```python
from build123d import *

# Parameters (mm, degrees)
F0_W      = 450
F0_H      = 450
F1_DEPTH  = 50
F2_W      = 40
F2_H      = 40
F3_DEPTH  = 400
F4_W      = 40
F4_H      = 40
F5_DEPTH  = 400
F6_W      = 40
F6_H      = 40
F7_DEPTH  = 400
F8_W      = 40
F8_H      = 40
F9_DEPTH  = 400
F10_W     = 450
F10_H     = 50
F11_DEPTH = 450
F13_DEPTH = 450
F15_DEPTH = 450.001
F17_DEPTH = 450.001
F18_DEPTH = 100
F19_DEPTH = 100
F20_DEPTH = 200
F21_DEPTH = 200


with BuildPart() as f1:
    # F0 (on Top) → F1 (new body)
    with BuildSketch(Plane.XY):
        with Locations((225, 225)):
            Rectangle(F0_W, F0_H)
    extrude(amount=F1_DEPTH)

    # F2 (on face) → F3 (join)
    with BuildSketch(Plane(origin=(0, 0, 0), x_dir=(1, 0, 0), z_dir=(0, 0, -1))):
        with Locations((20, -430)):
            Rectangle(F2_W, F2_H)
    extrude(amount=F3_DEPTH)

    # F4 (on face) → F5 (join)
    with BuildSketch(Plane(origin=(0, 0, 0), x_dir=(1, 0, 0), z_dir=(0, 0, -1))):
        with Locations((20, -20)):
            Rectangle(F4_W, F4_H)
    extrude(amount=F5_DEPTH)

    # F6 (on face) → F7 (join)
    with BuildSketch(Plane(origin=(0, 0, 0), x_dir=(1, 0, 0), z_dir=(0, 0, -1))):
        with Locations((430, -430)):
            Rectangle(F6_W, F6_H)
    extrude(amount=F7_DEPTH)

    # F8 (on face) → F9 (join)
    with BuildSketch(Plane(origin=(0, 0, 0), x_dir=(1, 0, 0), z_dir=(0, 0, -1))):
        with Locations((430, -20)):
            Rectangle(F8_W, F8_H)
    extrude(amount=F9_DEPTH)

    # F10 (on face) → F11 (join)
    with BuildSketch(Plane.XY.offset(50)):
        with Locations((225, 425)):
            Rectangle(F10_W, F10_H)
    extrude(amount=F11_DEPTH)

    # F12 (on face) → F13 (cut)
    with BuildSketch(Plane.YZ.offset(450)):
        Polygon((400, 500), (400, 50), (430, 500), align=None)
    extrude(amount=-F13_DEPTH, mode=Mode.SUBTRACT)

    # F14 (on face) → F15 (cut, through all)
    with BuildSketch(Plane(origin=(0, 0, 0), x_dir=(0, -1, 0), z_dir=(-1, 0, 0))):
        Polygon((-410, -400), (-410, 0), (-430, -400), align=None)
    extrude(amount=-F15_DEPTH, mode=Mode.SUBTRACT)

    # F16 (on face) → F17 (cut, through all)
    with BuildSketch(Plane(origin=(0, 0, 0), x_dir=(0, -1, 0), z_dir=(-1, 0, 0))):
        Polygon((-20, -400), (-40, 0), (-40, -400), align=None)
    extrude(amount=-F17_DEPTH, mode=Mode.SUBTRACT)

    # F18 (add): a face of the model
    f18_faces = [f1.faces().sort_by_distance(p)[0] for p in [
        (225, 200, 50),
    ]]
    extrude(f18_faces, amount=F18_DEPTH)

    # F19 (cut): a face of the model
    f19_faces = [f1.faces().sort_by_distance(p)[0] for p in [
        (225, 200, 150),
    ]]
    extrude(f19_faces, amount=-F19_DEPTH, mode=Mode.SUBTRACT)

    # F20 (add): a face of the model
    f20_faces = [f1.faces().sort_by_distance(p)[0] for p in [
        (225, 200, 50),
    ]]
    extrude(f20_faces, amount=F20_DEPTH)

    # F21 (cut): a face of the model
    f21_faces = [f1.faces().sort_by_distance(p)[0] for p in [
        (225, 200, 250),
    ]]
    extrude(f21_faces, amount=-F21_DEPTH, mode=Mode.SUBTRACT)


solid = f1.part
```
Verification items for the finished model (mm, model axes). A direction names the side the tool comes from. Round coordinates to 2 decimals unless told otherwise and drop trailing zeros. Write each loop counter-clockwise with the first axis right and the second up, starting at its lowest first coordinate (ties: lowest second). Pieces come first, ordered by that corner, then holes. Notation, with made-up numbers: (4, -11) -> (32, -11) arc R13 ccw to (32, 8) -> close; hole circle Ø4 at (-31.75, -13.75). An arc over 180 degrees is marked (long way). Write each question's results on one line, items separated by ' | '. Start each with the question number.
1. Set-up check for faces 4 (the flat face through (222, 203, 50)), 5 (the flat face through (410, 16, -197)), 6 (the flat face through (19.72, 419.86, -197.2)), 7 (the flat face through (222, 228, 0)): record each of +Z, -Z, +X, -X, +Y, -Y from which the full face is reachable in a straight line by a thin tool's end or side.
2. Material ranges on probe 1 along Z at (x, y) = (359.5, 210); probe 2 along Y at (x, z) = (129.5, 81); probe 3 along Y at (x, z) = (85, 101), recorded low to high. Write a range as from..to.
3. Cross-section at A-A (z = -174). Enter the section's corners in (x, y), then the cut area to 3 significant figures.
4. Cross-section at D-D (z = 413). Enter the section's corners in (x, y), then the cut area to 3 significant figures.
5. Cross-section at B-B (y = 31). Enter the section's corners in (x, z).
6. Draft check along Y on faces 1 (the flat face through (429.72, 29.86, -202.8)), 2 (the flat face through (450, 257, 15)), 3 (the flat face through (241, 0, 7)). Enter one of: +Y half, -Y half, draft (parallel to the pull), parting line (faces both ways), or undercut.
7. Depth check by flat-ended pin: P1, Ø1.5, axis at x = 340.5, y = 84, coming from the +Z side. Enter the tip coordinate at first touch or a pass-through.
8. Cross-section at C-C (x = 104). Enter the section's corners in (y, z).
Solutions:
1) face 4: +Z, +X, -X, -Y | face 5: -Z, +Y, -Y | face 6: -Z, +X, -X | face 7: -Z
2) probe 1: z = 0..50 | probe 2: y = 402.07..450 | probe 3: y = 403.4..450
3) outline: (0, 0) -> (40, 0) -> (40, 31.3) -> (0, 31.3) -> close; (0, 418.7) -> (40, 418.7) -> (40, 450) -> (0, 450) -> close; (410, 0) -> (450, 0) -> (450, 31.3) -> (410, 31.3) -> close; (410, 418.7) -> (450, 418.7) -> (450, 450) -> (410, 450) -> close | area: 5,010 mm2
4) outline: (0, 424.2) -> (450, 424.2) -> (450, 450) -> (0, 450) -> close | area: 11,600 mm2
5) outline: (0, -180) -> (40, -180) -> (40, 0) -> (410, 0) -> (410, -180) -> (450, -180) -> (450, 50) -> (0, 50) -> close
6) face 1: undercut | face 2: draft | face 3: -Y half
7) P1: stops at z = 50
8) outline: (0, 0) -> (450, 0) -> (450, 500) -> (430, 500) -> (400, 50) -> (0, 50) -> close
